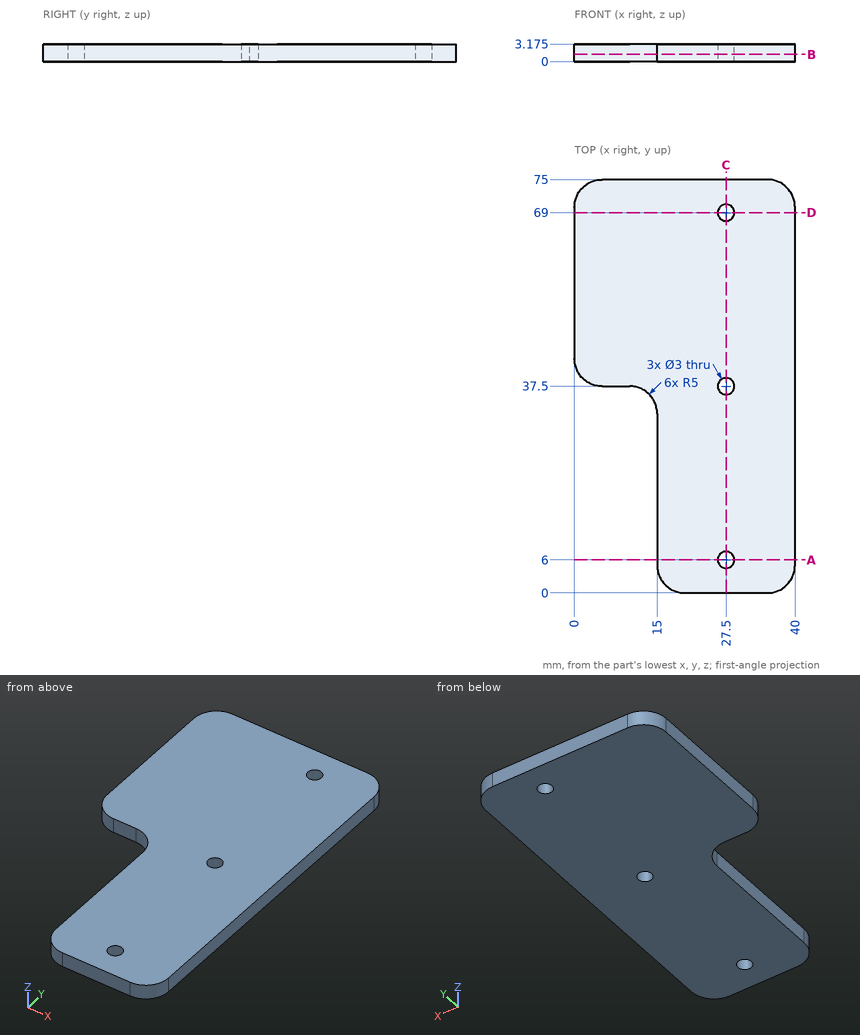
Geometry check sheet. Reference: drawing and pictorial views, mm from the part's lowest x, y, z. Round coordinates to 2 decimals unless told otherwise and drop trailing zeros. Write each loop counter-clockwise with the first axis right and the second up, starting at its lowest first coordinate (ties: lowest second). Pieces come first, ordered by that corner, then holes. Notation, with made-up numbers: (80, 81.5) -> (90, 81.5) arc R13 ccw to (90, 85.5) -> close; hole circle Ø7 at (70.5, -38.5). An arc over 180 degrees is marked (long way). Put each result on its own line as item: value.
1) Cross-section at A-A, the plane y = 6. Enter the section's corners in (x, z) (3 decimals), plus the area to 4 significant figures.
Recorded:
outline: (15, 0) -> (26, 0) -> (26, 3.175) -> (15, 3.175) -> close; (29, 0) -> (40, 0) -> (40, 3.175) -> (29, 3.175) -> close
area: 69.85 mm2
2) Depth check by flat-ended pin: P1, Ø1.6, axis at x = 8.5, z = 1, coming from the -Y side. Enter the tip coordinate at first touch or a pass-through.
Recorded:
P1: stops at y = 37.5
3) Thickness scan on probe 1 along Y at (x, z) = (27.5, 1.95); probe 2 along X at (y, z) = (69, 1.55); probe 3 along Y at (x, z) = (26.5, 2.1). Record the ranges inside material, lowest first. Write a range as from..to.
Recorded:
probe 1: y = 0..4.5, 7.5..36, 39..67.5, 70.5..75
probe 2: x = 0..26, 29..40
probe 3: y = 0..4.88, 7.12..36.38, 38.62..67.88, 70.12..75
4) Cross-section at B-B, the plane z = 1.3. Enter the section's corners in (x, y), plus the area to 3 significant figures.
Recorded:
outline: (0, 42.5) arc R5 ccw to (5, 37.5) -> (10, 37.5) arc R5 cw to (15, 32.5) -> (15, 5) arc R5 ccw to (20, 0) -> (35, 0) arc R5 ccw to (40, 5) -> (40, 70) arc R5 ccw to (35, 75) -> (5, 75) arc R5 ccw to (0, 70) -> close; hole circle Ø3 at (27.5, 6); hole circle Ø3 at (27.5, 37.5); hole circle Ø3 at (27.5, 69)
area: 2,390 mm2
5) Cross-section at D-D, the plane y = 69. Enter the section's corners in (x, z) (3 decimals), plus the area to 3 significant figures.
Recorded:
outline: (0, 0) -> (26, 0) -> (26, 3.175) -> (0, 3.175) -> close; (29, 0) -> (40, 0) -> (40, 3.175) -> (29, 3.175) -> close
area: 117 mm2
6) Cross-section at C-C, the plane x = 27.5. Enter the section's corners in (y, z) (3 decimals).
Recorded:
outline: (0, 0) -> (4.5, 0) -> (4.5, 3.175) -> (0, 3.175) -> close; (7.5, 0) -> (36, 0) -> (36, 3.175) -> (7.5, 3.175) -> close; (39, 0) -> (67.5, 0) -> (67.5, 3.175) -> (39, 3.175) -> close; (70.5, 0) -> (75, 0) -> (75, 3.175) -> (70.5, 3.175) -> close
